Check sheet for the modelled part. Datum: model origin and axes. Units: mm. A direction names the side the tool comes from. Round coordinates to 2 decimals unless told otherwise and drop trailing zeros. Write each loop counter-clockwise with the first axis right and the second up, starting at its lowest first coordinate (ties: lowest second). Pieces come first, ordered by that corner, then holes. Notation, with made-up numbers: M 75.5,53.25 L 127.5,53.25 A22 cw 127.5,64.25 Z; hole C -14,63 d6. An arc over 180 degrees is marked long. Answer in a Markdown table with one row per item.
```python
from build123d import *

# Parameters (mm, degrees)
SKETCH1_R           = 2.15
BOSS_EXTRUDE1_DEPTH = 6
SKETCH3_R           = 2.15
BOSS_EXTRUDE2_DEPTH = 13.9
FILLET1_R           = 5
FILLET2_R           = 5
CHAMFER1_SIZE       = 0.5
CHAMFER1_SIZE2      = 0.866025404
FILLET3_R           = 0.5
FILLET4_R           = 2
FILLET5_R           = 0.5


with BuildPart() as part:
    # Sketch1 → Boss-Extrude1 (new body)
    with BuildSketch(Plane.XY):
        Polygon((-110, -8), (110, -8), (110, 8), (-110, 8), (-125, 5), (-125, -5), align=None)
        with Locations((-119, 0)):
            Circle(SKETCH1_R, mode=Mode.SUBTRACT)
        with BuildLine():
            Line((101.75, -2.25), (-77.75, -2.25))
            ThreePointArc((-77.75, -2.25), (-80, 0), (-77.75, 2.25))
            Line((-77.75, 2.25), (101.75, 2.25))
            ThreePointArc((101.75, 2.25), (104, 0), (101.75, -2.25))
        make_face(mode=Mode.SUBTRACT)
    extrude(amount=BOSS_EXTRUDE1_DEPTH)

    # Sketch3 → Boss-Extrude2 (add)
    with BuildSketch(Plane.XY.offset(6)):
        Polygon((-125, 5), (-125, -5), (-113, -7.4), (-113, 7.4), align=None)
        with Locations((-119, 0)):
            Circle(SKETCH3_R, mode=Mode.SUBTRACT)
    extrude(amount=BOSS_EXTRUDE2_DEPTH)

    # Fillet1
    fillet1_edges = [part.edges().sort_by_distance(p)[0] for p in [
        (110, 8, 3),
        (110, -8, 3),
    ]]
    fillet(fillet1_edges, radius=FILLET1_R)

    # Fillet2
    fillet2_edges = [part.edges().sort_by_distance(p)[0] for p in [
        (-125, -5, 9.95),
        (-125, 5, 9.95),
        (-113, 7.4, 12.95),
        (-113, -7.4, 12.95),
    ]]
    fillet(fillet2_edges, radius=FILLET2_R)

    # Chamfer1
    chamfer1_edges = [part.edges().sort_by_distance(p)[0] for p in [
        (-115.490290338, 6.901941932, 0),
        (-2.5, 8, 0),
        (-2.5, -8, 0),
        (12, -2.25, 0),
        (104, 0, 0),
        (12, 2.25, 0),
        (-80, 0, 0),
        (110, 0, 0),
        (108.535533906, 6.535533906, 0),
        (108.535533906, -6.535533906, 0),
        (-115.490290338, -6.901941932, 0),
        (-125, 0, 0),
        (-123.866710707, 4.070925014, 0),
        (-123.866710707, -4.070925014, 0),
    ]]
    chamfer1_side = [part.faces().sort_by_distance(p)[0] for p in [
        (-115.028350448, -4.592242485, 0),
    ]]
    chamfer(chamfer1_edges, length=CHAMFER1_SIZE, length2=CHAMFER1_SIZE2, reference=chamfer1_side[0])

    # Fillet3
    fillet3_edges = [part.edges().sort_by_distance(p)[0] for p in [
        (12, 2.25, 6),
        (104, 0, 6),
        (12, -2.25, 6),
        (-2.5, -8, 6),
        (-2.5, 8, 6),
        (110, 0, 6),
        (108.535533906, 6.535533906, 6),
        (108.535533906, -6.535533906, 6),
        (-80, 0, 6),
    ]]
    fillet(fillet3_edges, radius=FILLET3_R)

    # Fillet4
    fillet4_edges = [part.edges().sort_by_distance(p)[0] for p in [
        (-113, 0, 6),
        (-114.830055472, -5.167691193, 6),
        (-114.830055472, 5.167691193, 6),
    ]]
    fillet(fillet4_edges, radius=FILLET4_R)

    # Fillet5
    fillet5_edges = [part.edges().sort_by_distance(p)[0] for p in [
        (-113, 0, 19.9),
        (-119.980580676, -6.003883865, 19.9),
        (-119.980580676, 6.003883865, 19.9),
        (-125, 0, 19.9),
        (-123.866710707, 4.070925014, 19.9),
        (-123.866710707, -4.070925014, 19.9),
        (-114.830055472, 5.167691193, 19.9),
        (-114.830055472, -5.167691193, 19.9),
    ]]
    fillet(fillet5_edges, radius=FILLET5_R)


solid = part.part
```
1. Section check B-B, the plane z = 16.25. Record the cut outline in (x, y).
Found:
| item | result |
|---|---|
| outline | M -125,-0.9 A5 ccw -120.98,-5.8 L -118.98,-6.2 A5 ccw -113,-1.3 L -113,1.3 A5 ccw -118.98,6.2 L -120.98,5.8 A5 ccw -125,0.9 Z; hole C -119,0 d4.3 |
2. Access from +Z, -Z, +X, -X, +Y, -Y to the whole of each face (thin tool, end or side, straight path). Record for faces 5 (the face through (-4, -8, 3)), 6 (the face through (11, 2.25, 3)).
Found:
| item | result |
|---|---|
| face 5 | +Z, -Z, +X, -X, -Y |
| face 6 | +Z, -Z |
3. Go/stop test with flat-tipped pins: pin 1 (4 mm diameter, centred on y = 5.5, z = 5, fed in from +X); pin 2 (4 mm diameter, centred on y = 5.5, z = 13.5, fed in from -X); pin 3 (1.5 mm diameter, centred on y = 4, z = 7, fed in from +X); pin 4 (5 mm diameter, centred on x = -119, y = 0, fed in from -Z). Record where each tip stops, or that it passes through.
Found:
| item | result |
|---|---|
| pin 1 | stops at x = 109.97 |
| pin 2 | stops at x = -124.27 |
| pin 3 | stops at x = -112.56 |
| pin 4 | stops at z = 0 |
4. Section check A-A, the plane x = -15. Record the cut outline in (y, z).
Found:
| item | result |
|---|---|
| outline | M -8,0.87 L -7.5,0 L -2.75,0 L -2.25,0.87 L -2.25,5.5 A0.5 ccw -2.75,6 L -7.5,6 A0.5 ccw -8,5.5 Z; M 2.25,0.87 L 2.75,0 L 7.5,0 L 8,0.87 L 8,5.5 A0.5 ccw 7.5,6 L 2.75,6 A0.5 ccw 2.25,5.5 Z |
5. Draft check along Y on faces 1 (the face through (-123.562, 3.879, 0.247)), 2 (the face through (13, -2.25, 3)), 3 (the face through (-123.836, -4.108, 10.263)), 4 (the face through (-116.6, 0.1, 19.9)). Enter one of: +Y half, -Y half, draft (parallel to the pull), parting line (faces both ways), or undercut.
Found:
| item | result |
|---|---|
| face 1 | +Y half |
| face 2 | undercut |
| face 3 | -Y half |
| face 4 | draft |
6. Scan lines: L1, parallel to Y at x = -119, z = 11.75; L2, parallel to Y at x = 23.5, z = 3; L3, parallel to X at y = 1.5, z = 1. Record each from-to range of solid material in increasing order.
Found:
| item | result |
|---|---|
| L1 | y = -6.2 to -2.15, 2.15 to 6.2 |
| L2 | y = -8 to -2.25, 2.25 to 8 |
| L3 | x = -124.96 to -120.54, -117.46 to -79.43, 103.43 to 110 |
